```python
from build123d import *

# Parameters (mm, degrees)
SKETCH_1_W           = 67
SKETCH_1_H           = 118
EXTRUDE_1_DEPTH      = 32
SHELL_2_T            = -5
SKETCH_2_W           = 42
SKETCH_2_H           = 75
CUT_EXTRUDE_1_DEPTH  = 5
SKETCH_4_W           = 31
SKETCH_4_H           = 40
CUT_EXTRUDE_2_DEPTH  = 5
SKETCH_7_R           = 1.4
SKETCH_7_R_2         = 1.7
CUT_EXTRUDE_4_DEPTH  = 95.836701756
SKETCH_9_W           = 32
SKETCH_9_H           = 17
CUT_EXTRUDE_6_DEPTH  = 95.836701756
SKETCH_10_W          = 90
SKETCH_10_H          = 101
SKETCH_10_R          = 1.7
SKETCH_10_W_2        = 42
SKETCH_10_H_2        = 75
EXTRUDE_4_DEPTH      = 5
FILLET_5_R           = 10
FILLET_6_R           = 5
FILLET_10_R          = 1
CUT_EXTRUDE_7_DEPTH  = 10
SKETCH_14_W          = 10.7
SKETCH_14_H          = 101
SKETCH_14_W_2        = 12.3
CUT_EXTRUDE_8_DEPTH  = 80.420652226
FILLET_11_R          = 5
SKETCH_17_R          = 1.7
EXTRUDE_8_DEPTH      = 15
EXTRUDE_8_2_DEPTH    = 15
SKETCH_18_R          = 3
CUT_EXTRUDE_9_DEPTH  = 5
SKETCH_19_W          = 67
SKETCH_19_H          = 14.7
EXTRUDE_9_DEPTH      = 60
SKETCH_21_W          = 11.7
SKETCH_21_H          = 50
CUT_EXTRUDE_10_DEPTH = 60
SKETCH_22_R          = 1.7
CUT_EXTRUDE_11_DEPTH = 60
SKETCH_23_R          = 3
CUT_EXTRUDE_12_DEPTH = 4
SKETCH_24_W          = 35.6
SKETCH_24_H          = 51
CUT_EXTRUDE_13_DEPTH = 115.733125196
FILLET_14_R          = 5
FILLET_15_R          = 10
FILLET_16_R          = 20


with BuildPart() as part:
    # Sketch 1 → Extrude 1 (new body)
    with BuildSketch(Plane.XY):
        Rectangle(SKETCH_1_W, SKETCH_1_H)
    extrude(amount=EXTRUDE_1_DEPTH)

    # Shell 2
    shell_2_openings = [part.faces().sort_by_distance(p)[0] for p in [
        (0, 0, 32),
    ]]
    offset(amount=SHELL_2_T, openings=shell_2_openings, kind=Kind.INTERSECTION)

    # Sketch 2 → Cut-Extrude 1 (cut)
    with BuildSketch(Plane(origin=(0, 0, 0), x_dir=(-1, 0, 0), z_dir=(0, 0, -1))):
        with Locations((-0.8, 6.8)):
            Rectangle(SKETCH_2_W, SKETCH_2_H)
    extrude(amount=-CUT_EXTRUDE_1_DEPTH, mode=Mode.SUBTRACT)

    # Sketch 4 → Cut-Extrude 2 (cut)
    with BuildSketch(Plane.ZY.offset(33.5)):
        with Locations((16.5, -3)):
            Rectangle(SKETCH_4_W, SKETCH_4_H)
    extrude(amount=-CUT_EXTRUDE_2_DEPTH, mode=Mode.SUBTRACT)

    # Sketch 7 → Cut-Extrude 4 (cut, through all)
    with BuildSketch(Plane.ZY.offset(33.5)):
        with Locations((29.5, 44)):
            Circle(SKETCH_7_R)
        with Locations((29.5, -31)):
            Circle(SKETCH_7_R_2)
    extrude(amount=-CUT_EXTRUDE_4_DEPTH, mode=Mode.SUBTRACT)

    # Sketch 9 → Cut-Extrude 6 (cut, through all)
    with BuildSketch(Plane.ZY.offset(33.5)):
        with Locations((16, -50.5)):
            Rectangle(SKETCH_9_W, SKETCH_9_H)
    extrude(amount=-CUT_EXTRUDE_6_DEPTH, mode=Mode.SUBTRACT)

    # Sketch 10 → Extrude 4 (add)
    with BuildSketch(Plane.XY.offset(5)):
        with Locations((0.8, 8.5)):
            Rectangle(SKETCH_10_W, SKETCH_10_H)
        with Locations((39.8, 39.3)):
            Circle(SKETCH_10_R, mode=Mode.SUBTRACT)
        with Locations(Location((39.8, -25.7, 0), (0, 0, 180))):
            Circle(SKETCH_10_R, mode=Mode.SUBTRACT)
        with Locations((-38.2, -25.7)):
            Circle(SKETCH_10_R, mode=Mode.SUBTRACT)
        with Locations(Location((-38.2, 39.3, 0), (0, 0, 180))):
            Circle(SKETCH_10_R, mode=Mode.SUBTRACT)
        with Locations((0.8, 6.8)):
            Rectangle(SKETCH_10_W_2, SKETCH_10_H_2, mode=Mode.SUBTRACT)
    extrude(amount=-EXTRUDE_4_DEPTH)

    # Fillet 5
    fillet_5_edges = [part.edges().sort_by_distance(p)[0] for p in [
        (-31, -23, 5),
        (-31, 17, 5),
    ]]
    fillet(fillet_5_edges, radius=FILLET_5_R)

    # Fillet 6
    fillet_6_edges = [part.edges().sort_by_distance(p)[0] for p in [
        (-31, 17, 32),
        (-31, -23, 32),
    ]]
    fillet(fillet_6_edges, radius=FILLET_6_R)

    # Fillet 10
    fillet_10_edges = [part.edges().sort_by_distance(p)[0] for p in [
        (-28.5, 30.5, 5),
        (-28.5, -27.5, 5),
        (28.5, 6, 5),
    ]]
    fillet(fillet_10_edges, radius=FILLET_10_R)

    # Sketch 13 → Cut-Extrude 7 (cut)
    with BuildSketch(Plane(origin=(33.5, 0, 0), x_dir=(0, 0, -1), z_dir=(1, 0, 0))):
        with BuildLine():
            Line((-24.5, 37.5), (-9.5, 37.5))
            ThreePointArc((-9.5, 37.5), (-7, 40), (-9.5, 42.5))
            Line((-9.5, 42.5), (-24.5, 42.5))
            ThreePointArc((-24.5, 42.5), (-27, 40), (-24.5, 37.5))
        make_face()
        with BuildLine():
            Line((-24.5, 26), (-9.5, 26))
            ThreePointArc((-9.5, 26), (-7, 28.5), (-9.5, 31))
            Line((-9.5, 31), (-24.5, 31))
            ThreePointArc((-24.5, 31), (-27, 28.5), (-24.5, 26))
        make_face()
        with BuildLine():
            Line((-24.5, -8.5), (-9.5, -8.5))
            ThreePointArc((-9.5, -8.5), (-7, -6), (-9.5, -3.5))
            Line((-9.5, -3.5), (-24.5, -3.5))
            ThreePointArc((-24.5, -3.5), (-27, -6), (-24.5, -8.5))
        make_face()
        with BuildLine():
            Line((-24.5, -20), (-9.5, -20))
            ThreePointArc((-9.5, -20), (-7, -17.5), (-9.5, -15))
            Line((-9.5, -15), (-24.5, -15))
            ThreePointArc((-24.5, -15), (-27, -17.5), (-24.5, -20))
        make_face()
        with BuildLine():
            Line((-24.5, 19.5), (-9.5, 19.5))
            ThreePointArc((-9.5, 19.5), (-7, 17), (-9.5, 14.5))
            Line((-9.5, 14.5), (-24.5, 14.5))
            ThreePointArc((-24.5, 14.5), (-27, 17), (-24.5, 19.5))
        make_face()
        with BuildLine():
            Line((-24.5, 8), (-9.5, 8))
            ThreePointArc((-9.5, 8), (-7, 5.5), (-9.5, 3))
            Line((-9.5, 3), (-24.5, 3))
            ThreePointArc((-24.5, 3), (-27, 5.5), (-24.5, 8))
        make_face()
        with BuildLine():
            Line((-24.5, -26.5), (-9.5, -26.5))
            ThreePointArc((-9.5, -26.5), (-7, -29), (-9.5, -31.5))
            Line((-9.5, -31.5), (-24.5, -31.5))
            ThreePointArc((-24.5, -31.5), (-27, -29), (-24.5, -26.5))
        make_face()
    extrude(amount=-CUT_EXTRUDE_7_DEPTH, mode=Mode.SUBTRACT)

    # Sketch 14 → Cut-Extrude 8 (cut, through all)
    with BuildSketch(Plane.XY.offset(5)):
        with Locations((-38.85, 8.5)):
            Rectangle(SKETCH_14_W, SKETCH_14_H)
        with Locations((39.65, 8.5)):
            Rectangle(SKETCH_14_W_2, SKETCH_14_H)
    extrude(amount=-CUT_EXTRUDE_8_DEPTH, mode=Mode.SUBTRACT)

    # Fillet 11
    fillet_11_edges = [part.edges().sort_by_distance(p)[0] for p in [
        (-31, -42, 32),
        (31, -42, 32),
    ]]
    fillet(fillet_11_edges, radius=FILLET_11_R)



with BuildPart() as body_2:
    # Sketch 17 → Extrude 8 (new body)
    with BuildSketch(Plane(origin=(0, 59, 0), x_dir=(1, 0, 0), z_dir=(0, 1, 0))):
        with BuildLine():
            Line((33.5, -32), (43.901244563, -21.203513926))
            ThreePointArc((43.901244563, -21.203513926), (46, -16), (43.901244563, -10.796486074))
            Line((43.901244563, -10.796486074), (33.5, 0))
            Line((33.5, 0), (33.5, -32))
        make_face()
        with Locations(Location((38.5, -16, 0), (0, 0, 180))):
            Circle(SKETCH_17_R, mode=Mode.SUBTRACT)
    extrude(amount=-EXTRUDE_8_DEPTH)


with BuildPart() as body_3:
    # Sketch 17 → Extrude 8 2 (new body)
    with BuildSketch(Plane(origin=(0, 59, 0), x_dir=(1, 0, 0), z_dir=(0, 1, 0))):
        with BuildLine():
            Line((-33.5, -32), (-33.5, 0))
            Line((-33.5, 0), (-43.901244563, -10.796486074))
            ThreePointArc((-43.901244563, -10.796486074), (-46, -16), (-43.901244563, -21.203513926))
            Line((-43.901244563, -21.203513926), (-33.5, -32))
        make_face()
        with Locations((-38.5, -16)):
            Circle(SKETCH_17_R, mode=Mode.SUBTRACT)
    extrude(amount=-EXTRUDE_8_2_DEPTH)


with BuildPart() as cut_extrude_9_tool:
    # Sketch 18 → Cut-Extrude 9 (new body)
    with BuildSketch(Plane.XZ.offset(-44)):
        with Locations((-38.5, 16)):
            Circle(SKETCH_18_R)
        with Locations((38.5, 16)):
            Circle(SKETCH_18_R)
    extrude(amount=-CUT_EXTRUDE_9_DEPTH)


with BuildPart() as body_2_1:
    add(body_2.part)

    # Cut-Extrude 9: cut by cut_extrude_9_tool
    add(cut_extrude_9_tool.part, mode=Mode.SUBTRACT)


with BuildPart() as body_3_1:
    add(body_3.part)

    # Cut-Extrude 9: cut by cut_extrude_9_tool
    add(cut_extrude_9_tool.part, mode=Mode.SUBTRACT)


with BuildPart() as part_1:
    add(part.part)

    add(body_2_1.part)  # Extrude 9 merges body 2

    add(body_3_1.part)  # Extrude 9 merges body 3
    # Sketch 19 → Extrude 9 (add)
    with BuildSketch(Plane(origin=(0, 0, 0), x_dir=(-1, 0, 0), z_dir=(0, 0, -1))):
        with Locations((0, 51.65)):
            Rectangle(SKETCH_19_W, SKETCH_19_H)
    extrude(amount=EXTRUDE_9_DEPTH)

    # Sketch 21 → Cut-Extrude 10 (cut)
    with BuildSketch(Plane.XZ.offset(-44.3)):
        with Locations((27.65, -35)):
            Rectangle(SKETCH_21_W, SKETCH_21_H)
        with Locations((-27.65, -35)):
            Rectangle(SKETCH_21_W, SKETCH_21_H)
    extrude(amount=-CUT_EXTRUDE_10_DEPTH, mode=Mode.SUBTRACT)

    # Sketch 22 → Cut-Extrude 11 (cut)
    with BuildSketch(Plane.XZ.offset(-44.3)):
        with Locations((27.65, -5)):
            Circle(SKETCH_22_R)
        with Locations((-27.65, -5)):
            Circle(SKETCH_22_R)
    extrude(amount=-CUT_EXTRUDE_11_DEPTH, mode=Mode.SUBTRACT)

    # Sketch 23 → Cut-Extrude 12 (cut)
    with BuildSketch(Plane.XZ.offset(-44.3)):
        with Locations((27.65, -5)):
            Circle(SKETCH_23_R)
        with Locations((-27.65, -5)):
            Circle(SKETCH_23_R)
    extrude(amount=-CUT_EXTRUDE_12_DEPTH, mode=Mode.SUBTRACT)

    # Sketch 24 → Cut-Extrude 13 (cut, through all)
    with BuildSketch(Plane.XZ.offset(-44.3)):
        with Locations((0, -29.5)):
            Rectangle(SKETCH_24_W, SKETCH_24_H)
    extrude(amount=-CUT_EXTRUDE_13_DEPTH, mode=Mode.SUBTRACT)

    # Fillet 14
    fillet_14_edges = [part_1.edges().sort_by_distance(p)[0] for p in [
        (-21.8, 51.65, -60),
        (21.8, 51.65, -60),
        (21.8, 51.65, -10),
        (33.5, 51.65, -10),
        (-33.5, 51.65, -10),
        (-21.8, 51.65, -10),
    ]]
    fillet(fillet_14_edges, radius=FILLET_14_R)

    # Fillet 15
    fillet_15_edges = [part_1.edges().sort_by_distance(p)[0] for p in [
        (17.8, 51.65, -4),
        (17.8, 51.65, -55),
        (-17.8, 51.65, -55),
        (-17.8, 51.65, -4),
    ]]
    fillet(fillet_15_edges, radius=FILLET_15_R)

    # Fillet 16
    # the kernel refuses this fillet: 20 mm, written as the material it adds along each edge
    with BuildSketch(Plane(origin=(-33.5, 59, 0), x_dir=(0.007697620119081404, 0, -0.9999703728833682), z_dir=(0, -1, 0))) as fillet_16_piece_1:
        with BuildLine():
            CenterArc((8.140232948, -19.845455055), FILLET_16_R, 97.127382881, 36.36338903)
            Line((-5.624521804, -5.335750488), (-7.000997279, -3.884780031))
            Line((-7.000997279, -3.884780031), (-1.376475475, 1.450970457))
            Line((-1.376475475, 1.450970457), (0.01539524, 1.999940746))
            ThreePointArc((0.01539524, 1.999940746), (5.015247105, 1.961452645), (5.410567123, 1.984545506))
            Line((5.410567123, 1.984545506), (5.658718562, 0))
        make_face()
    extrude(amount=14.7)
    with BuildSketch(Plane(origin=(33.5, 59, 0), x_dir=(-0.00769762011907516, 0, -0.9999703728833682), z_dir=(0, -1, 0))) as fillet_16_piece_2:
        with BuildLine():
            CenterArc((8.140232948, 19.845455055), FILLET_16_R, 226.509228089, 36.36338903)
            Line((-5.624521804, 5.335750488), (-7.000997279, 3.884780031))
            Line((-7.000997279, 3.884780031), (-1.376475475, -1.450970457))
            Line((-1.376475475, -1.450970457), (0.01539524, -1.999940746))
            ThreePointArc((0.01539524, -1.999940746), (5.015247105, -1.961452645), (5.410567123, -1.984545506))
            Line((5.410567123, -1.984545506), (5.658718562, 0))
        make_face()
    extrude(amount=14.7)


solid = part_1.part
```
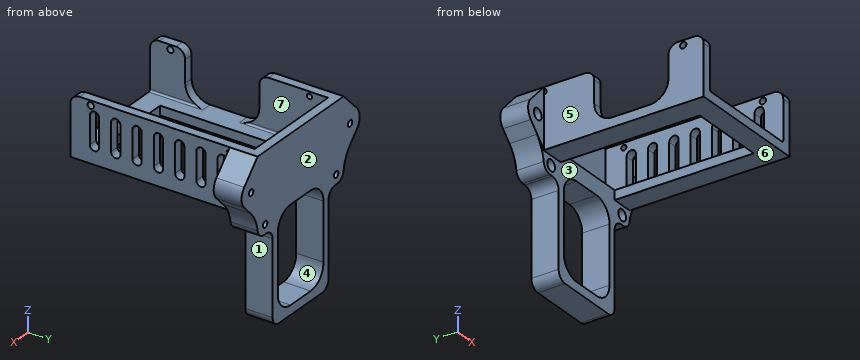
Read the model definition and answer for the solid it produces. Units are mm, in the model's axes. Face numbers are marked on the shaded views. A direction names the side the tool comes from. Round coordinates to 2 decimals unless told otherwise and drop trailing zeros. Loops run counter-clockwise (first coordinate to the right, second up) from the corner with the lowest first, then second, coordinate; pieces in that order, holes last. Notation, with made-up numbers: (57, 22.5) -> (104, 22.5) arc R23 ccw to (104, 36.5) -> close; hole circle Ø7 at (86, 45.5). An arc over 180 degrees is marked (long way). One line per item, written item: value.
1) A cutting plane is placed at B-B (y = 5.5). Determine the outline of the cut face in (x, z).
Answer list:
outline: (-33.5, 0) -> (-20.2, 0) -> (-20.2, 5) -> (-33.5, 5) -> close; (21.8, 0) -> (33.5, 0) -> (33.5, 7) -> (28.5, 7) -> (28.5, 6) arc R1 cw to (27.5, 5) -> (21.8, 5) -> close; (28.5, 27) -> (33.5, 27) -> (33.5, 32) -> (28.5, 32) -> close
2) Flat-ended cylindrical pins translate along their axes: P1, Ø6, axis at x = 20, y = 31, coming from the +Z side; P2, Ø5.5, axis at y = 19, z = 3.5, coming from the +X side; P3, Ø4, axis at x = 27.65, z = -5, coming from the -Y side. Find the tip coordinate at first contact, or state that the pin passes through.
Answer list:
P1: stops at z = 5
P2: stops at x = 33.5
P3: stops at y = 48.3
3) For the marked faces 4, 5, 6 and 7, determine the directions among +Z, -Z, +X, -X, +Y, -Y from which every point of the face is accessible in a straight line to the end or side of a thin tool.
Answer list:
face 4: +Y, -Y
face 5: +Z, -Z, -X, -Y
face 6: -Z, +X, -X, -Y
face 7: +Z, -Y
4) The mould has two halves that part along Y. Classify the marked faces 1, 2 and 3: pulls with the +Y half, pulls with the -Y half, needs draft (parallel to the pull), parting line crosses it, or undercut.
Answer list:
face 1: needs draft
face 2: pulls with the +Y half
face 3: undercut
5) A cutting plane is placed at A-A (z = -40). Determine the outline of the cut face in (x, y), and give its area (3 significant figures).
Answer list:
outline: (-21.8, 44.3) -> (-17.8, 44.3) -> (-17.8, 59) -> (-21.8, 59) -> close; (17.8, 44.3) -> (21.8, 44.3) -> (21.8, 59) -> (17.8, 59) -> close
area: 118 mm²
6) A cutting plane is placed at C-C (y = 23.5). Determine the outline of the cut face in (x, z), and give its area (3 significant figures).
Answer list:
outline: (-33.5, 0) -> (-20.2, 0) -> (-20.2, 5) -> (-27.5, 5) arc R1 cw to (-28.5, 6) -> (-28.5, 32) -> (-33.5, 32) -> close; (21.8, 0) -> (33.5, 0) -> (33.5, 32) -> (28.5, 32) -> (28.5, 6) arc R1 cw to (27.5, 5) -> (21.8, 5) -> close
area: 395 mm²
7) A cutting plane is placed at D-D (y = 40). Determine the outline of the cut face in (x, z).
Answer list:
outline: (-33.5, 0) -> (-20.2, 0) -> (-20.2, 5) -> (-27.5, 5) arc R1 cw to (-28.5, 6) -> (-28.5, 32) -> (-33.5, 32) -> close; (21.8, 0) -> (33.5, 0) -> (33.5, 7) -> (28.5, 7) -> (28.5, 6) arc R1 cw to (27.5, 5) -> (21.8, 5) -> close; (28.5, 27) -> (33.5, 27) -> (33.5, 32) -> (28.5, 32) -> close
8) Consider L1, parallel to Y at x = -31.1, z = 29.5; L2, parallel to Y at x = 21.5, z = 1; L3, parallel to Z at x = -27.65, y = 52.5. Determine where each line is inside the solid, lowest interval first. Write a range as [from, to].
Answer list:
L1: y = [-41.33, -32.7], [-29.3, -23.67], [17.67, 42.6], [45.4, 59]
L2: y = [-42, -30.7], [44.3, 59]
L3: z = [-10, -6.7], [-3.3, 5.01]
